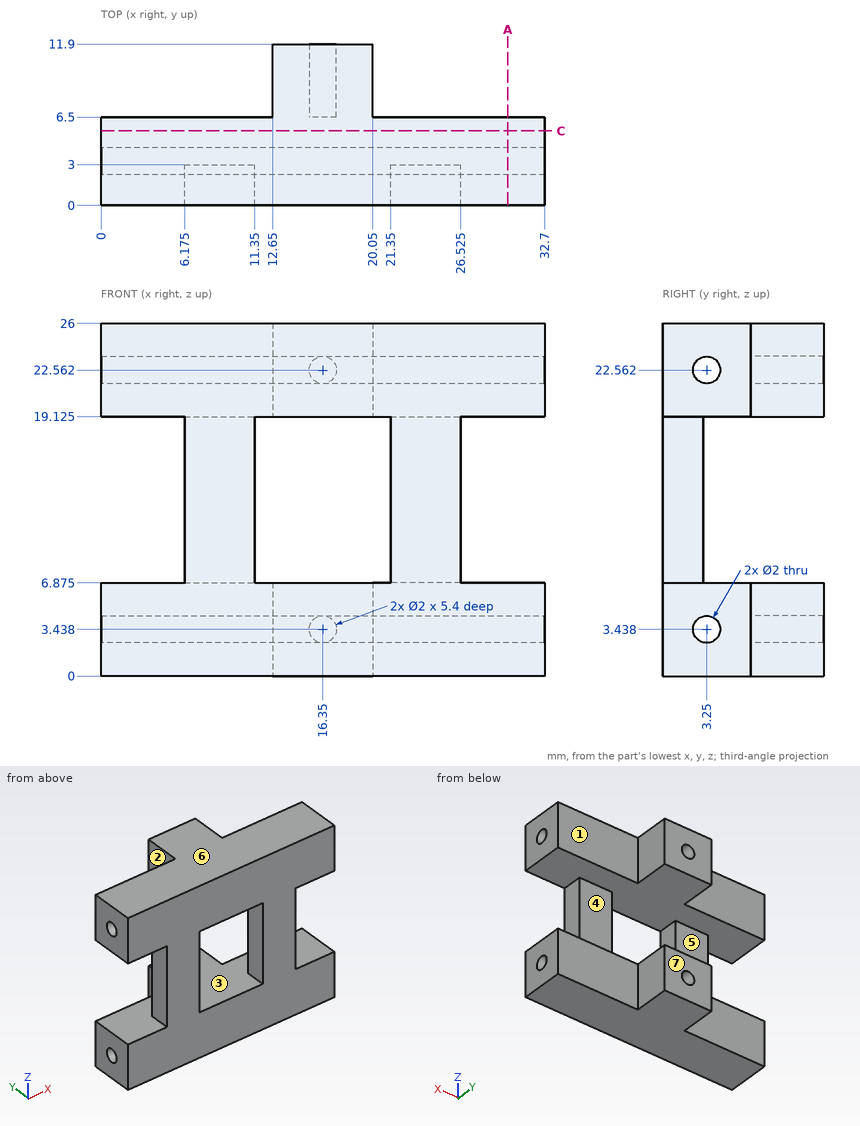
The drawing under review shows one solid part. Ordinate dimensions are in mm from its lowest x, y, z. A direction names the side the tool comes from. Coordinates: 2 decimals unless noted, no trailing zeros. Write each loop counter-clockwise with the first axis right and the second up, starting at its lowest first coordinate (ties: lowest second). Pieces come first, ordered by that corner, then holes. Notation, with made-up numbers: (68, -28.75) -> (124, -28.75) arc R18 ccw to (124, -21.75) -> close; hole circle Ø7 at (18, 86). An arc over 180 degrees is marked (long way). One line per item, written item: value. Start each with the question number.
Q1. Add section C-C, the plane y = 5.5. Give the boundary of the cut face in (x, z) (1 decimal).
Q2. To check wall thickness, follow probe 1 along Z at (x, y) = (16.35, 9.75) (1 decimal); probe 2 along Z at (x, y) = (20, 0.75) (1 decimal); probe 3 along Y at (x, z) = (14, 22.5). State the ranges of each line that lie inside material, in increasing order.
Q3. Clearance check with flat-ended pins moving along their axes: P1, Ø4.5, axis at y = 9.5, z = 22.5, coming from the +X side; P2, Ø3, axis at x = 16.35, z = 22.56, coming from the +Y side; P3, Ø2.5, axis at y = 10, z = 24, coming from the -X side; P4, Ø1.6, axis at x = 16.35, z = 3.44, coming from the +Y side. State where each tip first meets the part, or that it passes through.
Q4. The part is to be moulded in two halves that separate along Z. For the marked faces 5, 6 and 7, say which applies: +Z half, -Z half, draft (parallel to the pull), parting line (faces both ways), or undercut.
Q5. Add section A-A, the plane x = 30. Count the separate pieces of the cut face and the enclosed holes in it.
Q6. For the marked faces 1, 2, 3 and 4, list the 3-axis set-ups (+Z, -Z, +X, -X, +Y, -Y) from which the entire face can be reached by the end or side of a thin tool; tool diameter is ignored.
Response:
1. outline: (0, 0) -> (32.7, 0) -> (32.7, 6.9) -> (0, 6.9) -> close; (0, 19.1) -> (32.7, 19.1) -> (32.7, 26) -> (0, 26) -> close
2. probe 1: 0 to 2.4, 4.4 to 6.9, 19.1 to 21.6, 23.6 to 26
2. probe 2: 0 to 6.9, 19.1 to 26
2. probe 3: 0 to 2.25, 4.25 to 11.9
3. P1: x = 20.05
3. P2: y = 11.9
3. P3: x = 12.65
3. P4: y = 6.5
4. face 5: undercut
4. face 6: +Z half
4. face 7: draft
5. separate pieces: 2
5. enclosed holes: 2
6. face 1: +Z, -Z, +X, +Y
6. face 2: +Z, -Z, -X, +Y
6. face 3: +Y
6. face 4: +X, -X, +Y
